Design review of the part built by this model. Coordinates are the model's own, in mm. Give positions to 0.01 mm unless a question says otherwise; leave off trailing zeros. Order: outer loops, then holes, each group sorted by start corner. A loop starts at its lowest first (then second) coordinate and runs counter-clockwise, first axis right, second up.
```python
from build123d import *

# Parameters (mm, degrees)
F0_R            = 58.3586225364
F1_DEPTH        = 25.4
F3_DEPTH        = 25.401
F3_COPIES_COUNT = 28
F5_R            = 8.5203865575
F6_DEPTH        = 25.401
F7_T            = -2.54


# Not quite as in the source:
# - a feature of the source that left no trace in its solid (it failed there, or was rolled back) is left out
# - a pattern or mirror of a feature is missing from the dataset's text; its kind, count and spacing are read off the source's solid


with BuildPart() as f1:
    # F0 (on Front) → F1 (new body)
    with BuildSketch(Plane.XZ):
        Circle(F0_R)
    extrude(amount=F1_DEPTH)

    # F2 (on face) → F3 (cut, through all)
    with BuildSketch(Plane.XZ.offset(25.4)):
        with BuildLine():
            ThreePointArc((5.3432300873, 58.1134985746), (0, 58.3586225364), (-5.3432300873, 58.1134985746))
            ThreePointArc((-5.3432300873, 58.1134985746), (0, 53.0097727981), (5.3432300873, 58.1134985746))
        make_face()
    f3 = extrude(amount=-F3_DEPTH, mode=Mode.SUBTRACT)

    # F3_copies: F3 ×28 about axis
    f3_copies_axis = Axis((0, 0, 0), (0, 1, 0))
    for i in range(1, F3_COPIES_COUNT):
        add(f3.rotate(f3_copies_axis, i * 360 / F3_COPIES_COUNT), mode=Mode.SUBTRACT)

    # F5 (on face) → F6 (cut, through all)
    with BuildSketch(Plane.XZ.offset(25.4)):
        Circle(F5_R)
    extrude(amount=-F6_DEPTH, mode=Mode.SUBTRACT)

    # F7
    f7_openings = [f1.faces().sort_by_distance(p)[0] for p in [
        (0, 0, 51.366075),
    ]]
    offset(amount=F7_T, openings=f7_openings)


solid = f1.part
```
1. Take a section at A-A (x = 0). State the section outline as (y, z) points.
Recorded:
outline: (-25.4, -53.01) - (0, -53.01) - (0, -50.47) - (-22.86, -50.47) - (-22.86, -11.06) - (0, -11.06) - (0, -8.52) - (-25.4, -8.52) - close; (-25.4, 8.52) - (0, 8.52) - (0, 11.06) - (-22.86, 11.06) - (-22.86, 50.47) - (0, 50.47) - (0, 53.01) - (-25.4, 53.01) - close
2. Take a section at B-B (z = 0). State the section outline as (x, y) points, then the cut area to 3 significant figures.
Recorded:
outline: (-53.01, -25.4) - (-8.52, -25.4) - (-8.52, 0) - (-11.06, 0) - (-11.06, -22.86) - (-50.47, -22.86) - (-50.47, 0) - (-53.01, 0) - close; (8.52, -25.4) - (53.01, -25.4) - (53.01, 0) - (50.47, 0) - (50.47, -22.86) - (11.06, -22.86) - (11.06, 0) - (8.52, 0) - close
area: 458 mm2
3. Take a section at C-C (y = -5.25). State how many separate pieces and enclosed holes the cut face has, then the cut area to 3 significant figures.
Recorded:
separate pieces: 2
enclosed holes: 2
area: 1,330 mm2
4. For line 1 along Z through (x, y) = (-48.5, -9.25); line 2 along X through (y, z) = (-10, -10); line 3 along Z through (x, y) = (-6, -15.75), list the stretches that pass through material, from the lowest coordinate up.
Recorded:
line 1: z = -31.87 to -28.78, -21.86 to -18.57, 18.57 to 21.86, 28.78 to 31.87
line 2: x = -52.46 to -49.59, -4.73 to 4.73, 49.59 to 52.46
line 3: z = -58.05 to -53.23, -9.29 to -6.05, 6.05 to 9.29, 53.23 to 58.05
5. For pin 1 (5 mm diameter, centred on x = 13.5, z = 31, fed in from +Y); pin 2 (8 mm diameter, centred on y = -19.5, z = 36, fed in from -X); pin 3 (22 mm diameter, centred on x = 0, z = 0, fed in from +Y); pin 4 (2 mm diameter, centred on x = 18.5, y = -19, fed in from -Z), all flat-tipped, find the tip position at first contact; note any pin that passes through.
Recorded:
pin 1: stops at y = -22.86
pin 2: stops at x = -48.8
pin 3: stops at y = 0
pin 4: stops at z = -55.47
6. Take a section at D-D (x = -35). State the section outline as (y, z) points.
Recorded:
outline: (-25.4, -40.46) - (0, -40.46) - (0, -37.86) - (-22.86, -37.86) - (-22.86, 37.86) - (0, 37.86) - (0, 40.46) - (-25.4, 40.46) - close
7. Draft analysis for pull direction X (two halves, no side actions). For faces 1 (the face through (53.01, -12.88, 0.11)), 2 (the face through (-53.01, -12.88, -0.11)), 3 (the face through (10.55, -11.59, 3.32)), state which applies: pulls with the +X half, pulls with the -X half, needs draft (parallel to the pull), parting line crosses it, or undercut.
Recorded:
face 1: pulls with the +X half
face 2: pulls with the -X half
face 3: undercut
